Input: part model. Units: mm. Frame: model coordinates. Face numbers are marked on the shaded views. Round coordinates to 2 decimals unless told otherwise and drop trailing zeros. Write each loop counter-clockwise with the first axis right and the second up, starting at its lowest first coordinate (ties: lowest second). Pieces come first, ordered by that corner, then holes. Notation, with made-up numbers: (-37, -25.75) - (9, -25.75) arc R27 cw to (9, 0.25) - close; hole circle Ø5 at (-29.75, 58.25). An arc over 180 degrees is marked (long way). Use one line per item in the form item = value.
```python
from build123d import *

# Parameters (mm, degrees)
F0_W    = 2.54
F0_H    = 9.525
F2_SIZE = 0.3175
F3_SIZE = 0.9525
F4_W    = 2.263989
F4_H    = 4.7625


with BuildPart() as f1:
    # F0 (on Front) → F1 (revolve)
    with BuildSketch(Plane.XZ):
        with Locations((-12.3825, 0)):
            Rectangle(F0_W, F0_H)
    revolve(axis=Axis((0, 0, 0), (0, 0, -1)))

    # F2
    f2_edges = [f1.edges().sort_by_distance(p)[0] for p in [
        (11.1125, 0, 4.7625),
        (11.1125, 0, -4.7625),
    ]]
    chamfer(f2_edges, length=F2_SIZE)

    # F3
    f3_edges = [f1.edges().sort_by_distance(p)[0] for p in [
        (13.6525, 0, -4.7625),
        (13.6525, 0, 4.7625),
    ]]
    chamfer(f3_edges, length=F3_SIZE)

    # F4 (on Right) → F5 (revolve, cut)
    with BuildSketch(Plane.YZ):
        with Locations((13.831995, 0)):
            Rectangle(F4_W, F4_H)
    revolve(axis=Axis((0, 0, -0.389769), (0, 0, -1)), mode=Mode.SUBTRACT)


solid = f1.part
```
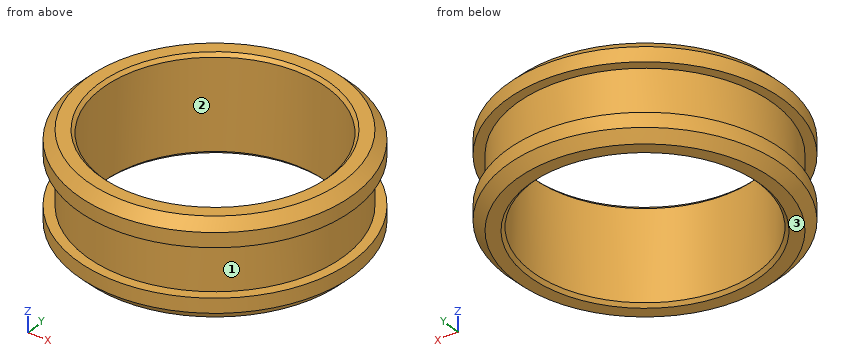
(1) Cut plane C-C on z = -1. Output: boundary loops of the cut face in (x, y) (1 decimal), then the cut area to 3 significant figures.
Derived:
outline = circle Ø25.4 at (0, 0); hole circle Ø22.2 at (0, 0)
area = 119 mm^2
(2) Material intervals for L1, parallel to Y at x = 9, z = 3.25; L2, parallel to X at y = -0.25, z = -2; L3, parallel to X at y = 3, z = 4.25, sorted ascending.
Derived:
L1 = -10.27 to -6.52, 6.52 to 10.27
L2 = -12.7 to -11.11, 11.11 to 12.7
L3 = -12.87 to -10.7, 10.7 to 12.87
(3) Cut plane A-A on x = 0. Output: boundary loops of the cut face in (y, z) (1 decimal).
Derived:
outline = (-13.7, -3.8) - (-12.7, -4.8) - (-11.4, -4.8) - (-11.1, -4.4) - (-11.1, 4.4) - (-11.4, 4.8) - (-12.7, 4.8) - (-13.7, 3.8) - (-13.7, 2.4) - (-12.7, 2.4) - (-12.7, -2.4) - (-13.7, -2.4) - close; (11.1, -4.4) - (11.4, -4.8) - (12.7, -4.8) - (13.7, -3.8) - (13.7, -2.4) - (12.7, -2.4) - (12.7, 2.4) - (13.7, 2.4) - (13.7, 3.8) - (12.7, 4.8) - (11.4, 4.8) - (11.1, 4.4) - close
(4) First-contact query: pin 1 Ø4 at (x, z) = (-7, -1.5) entering from +Y; pin 2 Ø2 at (x, z) = (1.5, 3) entering from -Y; pin 3 Ø5 at (y, z) = (4, 2) entering from -X. Flat tips, straight axial feed; report the tip coordinate or a pass-through.
Derived:
pin_1 = 12.62
pin_2 = -13.64
pin_3 = -13.57
(5) Draft query along Y for the marked faces 1, 2 and 3. Return one class per face: released by +Y, released by -Y, zero draft, split by the parting line, or undercut.
Derived:
face_1 = split by the parting line
face_2 = undercut
face_3 = zero draft
